Read the model definition and answer for the solid it produces. Units are mm, in the model's axes. A direction names the side the tool comes from. Coordinates: 2 decimals unless noted, no trailing zeros. Write each loop counter-clockwise with the first axis right and the second up, starting at its lowest first coordinate (ties: lowest second). Pieces come first, ordered by that corner, then holes. Notation, with made-up numbers: (-25.5, 7) -> (5.5, 7) arc R32 ccw to (5.5, 34) -> close; hole circle Ø1 at (63.25, -0.75). An arc over 180 degrees is marked (long way). Return JSON: item names as keys, results as strings.
from build123d import *

# Parameters (mm, degrees)
SKETCH_1_W          = 100
SKETCH_1_H          = 100
EXTRUDE_1_DEPTH     = 6
EXTRUDE_2_DEPTH     = 6
SKETCH_3_R          = 2.1
SKETCH_3_W          = 7
SKETCH_3_H          = 6
CUT_EXTRUDE_1_DEPTH = 7


with BuildPart() as part:
    # Эскиз1 → Бобышка-Вытянуть1 (new body)
    with BuildSketch(Plane.XY):
        Rectangle(SKETCH_1_W, SKETCH_1_H)
    extrude(amount=EXTRUDE_1_DEPTH)

    # Эскиз2 → Бобышка-Вытянуть2 (add)
    with BuildSketch(Plane.XY):
        with BuildLine():
            Line((13, 53), (-13, 53))
            ThreePointArc((-13, 53), (-14.118033989, 52.736067977), (-15, 52))
            Line((-15, 52), (-16.2, 50.4))
            ThreePointArc((-16.2, 50.4), (-16.552786405, 50.105572809), (-17, 50))
            Line((-17, 50), (17, 50))
            ThreePointArc((17, 50), (16.552786405, 50.105572809), (16.2, 50.4))
            Line((16.2, 50.4), (15, 52))
            ThreePointArc((15, 52), (14.118033989, 52.736067977), (13, 53))
        make_face()
    extrude(amount=EXTRUDE_2_DEPTH)

    # Эскиз3 → Вырез-Вытянуть1 (cut, through all)
    with BuildSketch(Plane.XY.offset(6)):
        with Locations((0, 47)):
            Circle(SKETCH_3_R)
        with Locations((9.531849908, 47)):
            Rectangle(SKETCH_3_W, SKETCH_3_H)
        with Locations((-9.531849908, 47)):
            Rectangle(SKETCH_3_W, SKETCH_3_H)
    extrude(amount=-CUT_EXTRUDE_1_DEPTH, mode=Mode.SUBTRACT)


solid = part.part
1. Consider L1, parallel to X at y = 46.5, z = 2.05; L2, parallel to Y at x = 0, z = 4.5; L3, parallel to Y at x = 10.5, z = 4.25. Determine where each line is inside the solid, lowest interval first.
Taken from the geometry:
{"L1": "x = -50 to -13.03, -6.03 to -2.04, 2.04 to 6.03, 13.03 to 50", "L2": "y = -50 to 44.9, 49.1 to 53", "L3": "y = -50 to 44, 50 to 53"}
2. The part is cut by section C-C (x = 0). Determine the outline of the cut face in (y, z).
Taken from the geometry:
{"outline": "(-50, 0) -> (44.9, 0) -> (44.9, 6) -> (-50, 6) -> close; (49.1, 0) -> (53, 0) -> (53, 6) -> (49.1, 6) -> close"}
3. For a pull along X with two mould halves and no side action, classify faces 6 (the face through (0, 53, 3)), 7 (the face through (50, -1, 3)), 8 (the face through (-13.032, 47, 3)) as +X half, -X half, draft (parallel to the pull), parting line (faces both ways), or undercut.
Taken from the geometry:
{"face 6": "draft", "face 7": "+X half", "face 8": "undercut"}
4. The part is cut by section B-B (z = 3.55). Determine the outline of the cut face in (x, y), then the cut area to 3 significant figures.
Taken from the geometry:
{"outline": "(-50, -50) -> (50, -50) -> (50, 50) -> (17, 50) arc R1 cw to (16.2, 50.4) -> (15, 52) arc R2.5 ccw to (13, 53) -> (-13, 53) arc R2.5 ccw to (-15, 52) -> (-16.2, 50.4) arc R1 cw to (-17, 50) -> (-50, 50) -> close; hole (-13.03, 44) -> (-6.03, 44) -> (-6.03, 50) -> (-13.03, 50) -> close; hole circle Ø4.2 at (0, 47); hole (6.03, 44) -> (13.03, 44) -> (13.03, 50) -> (6.03, 50) -> close", "area": "9,990 mm2"}
5. A tool of negligible diameter and unlimited length cuts with its end or side. For faces 1 (the face through (-34, 50, 3)), 2 (the face through (-6.032, 47, 3)), 3 (the face through (-1, 2, 0)), 4 (the face through (-1, 2, 6)), 5 (the face through (33, 50, 3)), from which of +Z, -Z, +X, -X, +Y, -Y can it reach the whole face along a straight path? Write none if from no direction.
Taken from the geometry:
{"face 1": "+Z, -Z, -X, +Y", "face 2": "+Z, -Z", "face 3": "-Z, +X, -X, +Y, -Y", "face 4": "+Z, +X, -X, +Y, -Y", "face 5": "+Z, -Z, +X, +Y"}
6. The part is cut by section A-A (y = 47). Determine the outline of the cut face in (x, z), then the cut area to 3 significant figures.
Taken from the geometry:
{"outline": "(-50, 0) -> (-13.03, 0) -> (-13.03, 6) -> (-50, 6) -> close; (-6.03, 0) -> (-2.1, 0) -> (-2.1, 6) -> (-6.03, 6) -> close; (2.1, 0) -> (6.03, 0) -> (6.03, 6) -> (2.1, 6) -> close; (13.03, 0) -> (50, 0) -> (50, 6) -> (13.03, 6) -> close", "area": "491 mm2"}
7. The part is cut by section D-D (x = -40). Determine the outline of the cut face in (y, z).
Taken from the geometry:
{"outline": "(-50, 0) -> (50, 0) -> (50, 6) -> (-50, 6) -> close"}
8. A flat-ended cylindrical pin translates along its axis: pin 1 Ø3 at (x, z) = (-28.5, 3.5) entering from +Y. Find the tip coordinate at first contact, or state that the pin passes through.
Taken from the geometry:
{"pin 1": "stops at y = 50"}
